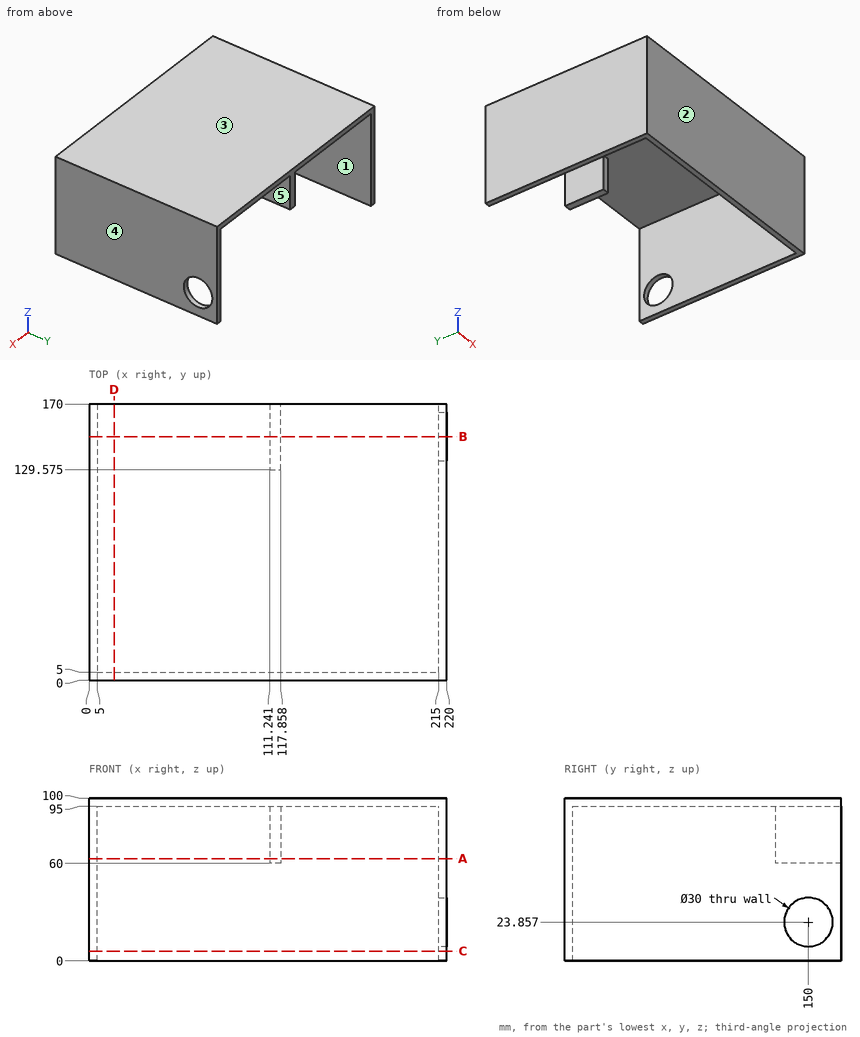
Source: three-view drawing plus pictorial views. Frame: mm from the lowest corner of the part. A direction names the side the tool comes from. Round coordinates to 2 decimals unless told otherwise and drop trailing zeros. Loops run counter-clockwise (first coordinate to the right, second up) from the corner with the lowest first, then second, coordinate; pieces in that order, holes last.
Item 1: Section B-B, the plane y = 150. Output: boundary loops of the cut face in (x, z), plus the area to 3 significant figures.
Checked values:
outline: (0, 0) - (5, 0) - (5, 95) - (111.24, 95) - (111.24, 60) - (117.86, 60) - (117.86, 95) - (215, 95) - (215, 38.86) - (220, 38.86) - (220, 100) - (0, 100) - close; (215, 0) - (220, 0) - (220, 8.86) - (215, 8.86) - close
area: 2,130 mm2
Item 2: Line query: L1, parallel to X at y = 143, z = 88.5; L2, parallel to X at y = 23.5, z = 79; L3, parallel to Y at x = 211, z = 20.5. Output: solid intervals per line, ascending.
Checked values:
L1: x = 0 to 5, 111.24 to 117.86, 215 to 220
L2: x = 0 to 5, 215 to 220
L3: y = 0 to 5
Item 3: Mould query, pull axis X, two halves, no side actions, for the marked faces 3, 4 and 5. Classes: released by +X, released by -X, zero draft, split by the parting line, or undercut.
Checked values:
face 3: zero draft
face 4: released by +X
face 5: undercut
Item 4: Section C-C, the plane z = 6. Output: boundary loops of the cut face in (x, y).
Checked values:
outline: (0, 0) - (220, 0) - (220, 170) - (215, 170) - (215, 5) - (5, 5) - (5, 170) - (0, 170) - close
Item 5: Section A-A, the plane z = 63. Output: boundary loops of the cut face in (x, y) (1 decimal).
Checked values:
outline: (0, 0) - (220, 0) - (220, 170) - (215, 170) - (215, 5) - (5, 5) - (5, 170) - (0, 170) - close; (111.2, 129.6) - (117.9, 129.6) - (117.9, 170) - (111.2, 170) - close
Item 6: Reachability of the marked faces 1 and 2 from +Z, -Z, +X, -X, +Y, -Y: full face, straight path, thin tool, end or side. Return the list, or none.
Checked values:
face 1: -Z, +Y
face 2: +Z, -Z, +X, -X, -Y
Item 7: Contact query for flat-ended pins moving along their axis: P1, Ø4, axis at x = 132.5, z = 65.5, coming from the +Y side; P2, Ø3.5, axis at x = 116, y = 158.5, coming from the -Z side; P3, Ø6, axis at x = 130.5, y = 114.5, coming from the -Z side. Output: stop coordinate, or through.
Checked values:
P1: stops at y = 5
P2: stops at z = 60
P3: stops at z = 95
Item 8: Section D-D, the plane x = 15.5. Output: boundary loops of the cut face in (y, z).
Checked values:
outline: (0, 0) - (5, 0) - (5, 95) - (170, 95) - (170, 100) - (0, 100) - close
